Source: CAD feature listing. Evaluate the final solid. Frame: model axes, mm. Coordinates: 2 decimals unless noted, no trailing zeros. Write each loop counter-clockwise with the first axis right and the second up, starting at its lowest first coordinate (ties: lowest second). Pieces come first, ordered by that corner, then holes. Notation, with made-up numbers: (87.25, 52) -> (129.25, 52) arc R25 cw to (129.25, 89) -> close; hole circle Ø3 at (-12.5, -6.5). An arc over 180 degrees is marked (long way). One line per item, written item: value. Start each with the question number.
1. Section query D-D, the plane z = -5. Output: boundary loops of the cut face in (x, y) (3 decimals).
2. First-contact query: P1, Ø4, axis at x = 586.5, z = -8, coming from the +Y side; P2, Ø3, axis at y = -1161.5, z = -7, coming from the +X side; P3, Ø5, axis at y = -939, z = -6.5, coming from the +X side. Flat tips, straight axial feed; report the tip coordinate or a pass-through.
3. Section query A-A, the plane x = 588.5. Output: boundary loops of the cut face in (y, z), and give its area (3 significant figures).
4. Line query: line 1 (Y direction, x = 515, z = -4.25); line 2 (X direction, y = -687, z = -2.25) (3 decimals); line 3 (Y direction, x = 905.5, z = -7.5). Output: solid intervals per line, ascending.
5. Section query C-C, the plane x = 1432.5. Output: boundary loops of the cut face in (y, z), and give its area (3 significant figures).
6. Section query B-B, the plane y = -1159. Output: boundary loops of the cut face in (x, z), and give its area (3 significant figures).
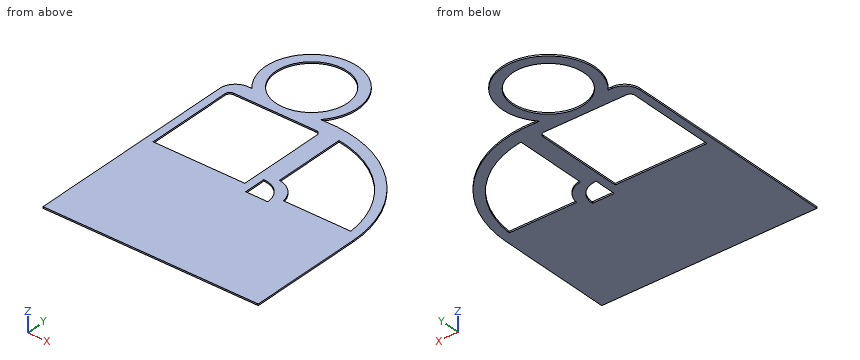
from build123d import *

# Parameters (mm, degrees)
SKETCH1_R           = 232.012436726
BOSS_EXTRUDE2_DEPTH = 10


with BuildPart() as part:
    # Sketch1 → Boss-Extrude2 (new body)
    with BuildSketch(Plane.XY):
        with BuildLine():
            Line((846.568769473, -512.108653834), (820.175567223, -512.108653834))
            ThreePointArc((820.175567223, -512.108653834), (596.568769473, -12.108653834), (372.961971723, -512.108653834))
            Line((372.961971723, -512.108653834), (346.568769473, -512.108653834))
            ThreePointArc((346.568769473, -512.108653834), (275.858091355, -541.397975715), (246.568769473, -612.108653834))
            Line((246.568769473, -612.108653834), (246.568769473, -1812.108653834))
            Line((246.568769473, -1812.108653834), (246.568769473, -2012.242939545))
            Line((246.568769473, -2012.242939545), (946.568769473, -2012.242939545))
            Line((946.568769473, -2012.242939545), (1646.568769473, -2012.242939545))
            Line((1646.568769473, -2012.242939545), (1646.568769473, -1812.108653834))
            Line((1646.568769473, -1812.108653834), (1646.568769473, -1262.242939545))
            ThreePointArc((1646.568769473, -1262.242939545), (1409.039966295, -713.90421061), (846.568769473, -512.108653834))
        make_face()
        with BuildLine():
            Line((946.568769473, -1260.416440178), (946.568769473, -1116.807153033))
            ThreePointArc((946.568769473, -1116.807153033), (1048.115870255, -1158.869339396), (1090.178056619, -1260.416440178))
            Line((1090.178056619, -1260.416440178), (946.568769473, -1260.416440178))
        make_face(mode=Mode.SUBTRACT)
        with BuildLine():
            ThreePointArc((298.257173598, -633.714224791), (307.043970163, -612.501021355), (328.257173598, -603.714224791))
            Line((328.257173598, -603.714224791), (864.880365349, -603.714224791))
            ThreePointArc((864.880365349, -603.714224791), (886.093568784, -612.501021355), (894.880365349, -633.714224791))
            Line((894.880365349, -633.714224791), (894.880365349, -1203.714224791))
            Line((894.880365349, -1203.714224791), (298.257173598, -1203.714224791))
            Line((298.257173598, -1203.714224791), (298.257173598, -633.714224791))
        make_face(mode=Mode.SUBTRACT)
        with Locations((596.568769473, -312.108653834)):
            Circle(SKETCH1_R, mode=Mode.SUBTRACT)
        with BuildLine():
            Line((1012.065009988, -1072.068666538), (1012.065009988, -600.862482616))
            ThreePointArc((1012.065009988, -600.862482616), (1405.330319639, -800.571245417), (1584.263077669, -1203.714224791))
            Line((1584.263077669, -1203.714224791), (1145.378172354, -1203.714224791))
            ThreePointArc((1145.378172354, -1203.714224791), (1101.465382273, -1114.859550352), (1012.065009988, -1072.068666538))
        make_face(mode=Mode.SUBTRACT)
    extrude(amount=-BOSS_EXTRUDE2_DEPTH)


solid = part.part
Computed values:
1. outline: (246.569, -2012.243) -> (1646.569, -2012.243) -> (1646.569, -1262.243) arc R751.688 ccw to (846.569, -512.109) -> (820.176, -512.109) arc R300 ccw (long way) to (372.962, -512.109) -> (346.569, -512.109) arc R100 ccw to (246.569, -612.109) -> close; hole (298.257, -1203.714) -> (894.88, -1203.714) -> (894.88, -633.714) arc R30 ccw to (864.88, -603.714) -> (328.257, -603.714) arc R30 ccw to (298.257, -633.714) -> close; hole circle Ø464.025 at (596.569, -312.109); hole (946.569, -1260.416) -> (1090.178, -1260.416) arc R143.609 ccw to (946.569, -1116.807) -> close; hole (1012.065, -1072.069) arc R151.742 cw to (1145.378, -1203.714) -> (1584.263, -1203.714) arc R658.332 ccw to (1012.065, -600.862) -> close
2. P1: stops at y = -12.22
2. P2: stops at x = 1639.99
2. P3: stops at x = 1574.7
3. outline: (-2012.24, -10) -> (-1203.71, -10) -> (-1203.71, 0) -> (-2012.24, 0) -> close; (-603.71, -10) -> (-543.98, -10) -> (-543.98, 0) -> (-603.71, 0) -> close; (-80.24, -10) -> (-12.22, -10) -> (-12.22, 0) -> (-80.24, 0) -> close
3. area: 9,360 mm²
4. line 1: y = -2012.24 to -1203.71, -603.71 to -529.31, -94.91 to -23.41
4. line 2: x = 246.569 to 298.257, 894.88 to 1012.065, 1262.736 to 1378.751
4. line 3: y = -2012.24 to -510.63
5. outline: (-2012.24, -10) -> (-1203.71, -10) -> (-1203.71, 0) -> (-2012.24, 0) -> close; (-831.03, -10) -> (-736.89, -10) -> (-736.89, 0) -> (-831.03, 0) -> close
5. area: 9,030 mm²
6. outline: (246.57, -10) -> (298.26, -10) -> (298.26, 0) -> (246.57, 0) -> close; (894.88, -10) -> (946.57, -10) -> (946.57, 0) -> (894.88, 0) -> close; (1048.25, -10) -> (1132.51, -10) -> (1132.51, 0) -> (1048.25, 0) -> close; (1579.31, -10) -> (1639.44, -10) -> (1639.44, 0) -> (1579.31, 0) -> close
6. area: 2,480 mm²
